Autodesk Inventor part; units mm, degrees
ref_plane "washer_to_base_XY" through (0, -0.48, 0) normal (0, 1, 0) x (1, 0, 0)
ref_plane "washer_to_base_YZ" through (0, -0.48, 0) normal (1, 0, 0) x (0, 0, -1)
ref_plane "washer_to_base_ZX" through (0, -0.48, 0) normal (0, 0, -1) x (0, 1, 0)
sketch "Sketch_1" plane through (0, 0, 0) normal (1, 0, 0) x (0, 1, 0)
  arc A0 (1.4, 9.75) -> (0, 8.35) centre (1.4, 8.35) ccw
  line L0 (0, 8.35) -> (0, -8.35)
  arc A1 (0, -8.35) -> (1.4, -9.75) centre (1.4, -8.35) ccw
  line L1 (1.4, -9.75) -> (16.2, -9.75)
  line L2 (16.2, -9.75) -> (16.2, -8.97)
  line L3 (16.2, -8.97) -> (0.7, -8.97)
  line L4 (0.7, -8.97) -> (0.7, 8.97)
  line L5 (0.7, 8.97) -> (16.2, 8.97)
  line L6 (16.2, 8.97) -> (16.2, 9.75)
  line L7 (16.2, 9.75) -> (1.4, 9.75)
extrude "Extrusion1" add sketch "Sketch_1" along normal mid plane 29.8667
sketch "Sketch_3" plane through (0, 0, 9.75) normal (0, 0, 1) x (1, 0, 0)
  line L0 (-22, 25) -> (-22, 0)
  line L1 (-22, 0) -> (-10.85, 0)
  line L2 (-10.85, 0) -> (-10.85, 0.7)
  line L3 (-10.85, 0.7) -> (-12.7818, 13.6261)
  arc A0 (-12.7301, 13.9322) -> (-12.7818, 13.6261) centre (-12.2873, 13.7) ccw
  line L4 (-12.7301, 13.9322) -> (-8.2588, 12.7341)
  arc A1 (-8.2588, 12.7341) -> (-7, 13.7) centre (-8, 13.7) ccw
  line L5 (-7, 13.7) -> (-7, 15.2)
  arc A2 (-5, 15.2) -> (-7, 15.2) centre (-6, 15.2) ccw
  line L6 (-5, 15.2) -> (-5, 0)
  line L7 (-5, 0) -> (5, 0)
  line L8 (5, 0) -> (5, 14.7)
  arc A3 (8, 14.7) -> (5, 14.7) centre (6.5, 14.7) ccw
  line L9 (8, 14.7) -> (8, 13.7)
  arc A4 (8, 13.7) -> (9.3545, 12.765) centre (9, 13.7) ccw
  line L10 (9.3545, 12.765) -> (13.1394, 14.2)
  arc A5 (13.6339, 13.6264) -> (13.1394, 14.2) centre (13.1394, 13.7) ccw
  line L11 (13.6339, 13.6264) -> (11.6047, 0)
  line L12 (11.6047, 0) -> (22, 0)
  line L13 (22, 0) -> (22, 25)
  line L14 (22, 25) -> (-22, 25)
extrude "Extrusion2" cut sketch "Sketch_3" against normal blind 1.4
sketch "Sketch_2" plane through (0, 0, -9.75) normal (0, 0, 1) x (1, 0, 0)
  line L0 (-22, 25) -> (-22, 0)
  line L1 (-22, 0) -> (-10.85, 0)
  line L2 (-10.85, 0) -> (-10.85, 0.7)
  line L3 (-10.85, 0.7) -> (-12.7818, 13.6261)
  arc A0 (-12.7301, 13.9322) -> (-12.7818, 13.6261) centre (-12.2873, 13.7) ccw
  line L4 (-12.7301, 13.9322) -> (-8.2588, 12.7341)
  arc A1 (-8.2588, 12.7341) -> (-7, 13.7) centre (-8, 13.7) ccw
  line L5 (-7, 13.7) -> (-7, 15.2)
  arc A2 (-5, 15.2) -> (-7, 15.2) centre (-6, 15.2) ccw
  line L6 (-5, 15.2) -> (-5, 0)
  line L7 (-5, 0) -> (5, 0)
  line L8 (5, 0) -> (5, 14.7)
  arc A3 (8, 14.7) -> (5, 14.7) centre (6.5, 14.7) ccw
  line L9 (8, 14.7) -> (8, 13.7)
  arc A4 (8, 13.7) -> (9.3545, 12.765) centre (9, 13.7) ccw
  line L10 (9.3545, 12.765) -> (13.1394, 14.2)
  arc A5 (13.6339, 13.6264) -> (13.1394, 14.2) centre (13.1394, 13.7) ccw
  line L11 (13.6339, 13.6264) -> (11.6047, 0)
  line L12 (11.6047, 0) -> (22, 0)
  line L13 (22, 0) -> (22, 25)
  line L14 (22, 25) -> (-22, 25)
extrude "Extrusion3" cut sketch "Sketch_2" along normal blind 1.4
sketch "Sketch4" plane through (-5, 0, 8.35) normal (0, -1, 0) x (1, 0, 0)
  point P0 (5, -8.35)
hole "Hole1" at (0, 0, 0) direction (0, 1, 0) diameter 10.5 depth 1
sketch "Sketch_5" plane through (0, 0, 0) normal (0, 0, 1) x (1, 0, 0)
  line L0 (-15.85, 1) -> (-15.85, -1)
  line L1 (-15.85, -1) -> (15.62, -1)
  line L2 (15.62, -1) -> (15.62, 1)
  line L3 (15.62, 1) -> (12.12, 1)
  line L4 (12.12, 1) -> (12.12, 0)
  line L5 (12.12, 0) -> (-10.85, 0)
  line L6 (-10.85, 0) -> (-10.85, 1)
  line L7 (-10.85, 1) -> (-15.85, 1)
extrude "Extrusion4" cut sketch "Sketch_5" along normal mid plane 16.7
sketch "Sketch_9" plane through (0, 0, 9.75) normal (0, 0, 1) x (1, 0, 0)
  line L0 (11.6047, 0) -> (22, 0)
  line L1 (22, 0) -> (22, 25)
  line L2 (22, 25) -> (15.3276, 25)
  line L3 (15.3276, 25) -> (11.6047, 0)
extrude "Extrusion5" cut sketch "Sketch_9" against normal blind 19.5
sketch "Sketch_6" plane through (-10.85, 0, 0) normal (1, 0, 0) x (0, 0, -1)
  arc A0 (-8.265, -7.8) -> (-6.765, -9.3) centre (-6.765, -7.8) ccw
  line L0 (-6.765, -9.3) -> (6.765, -9.3)
  arc A1 (6.765, -9.3) -> (8.265, -7.8) centre (6.765, -7.8) ccw
  line L1 (8.265, -7.8) -> (8.265, 0.7)
  line L2 (8.265, 0.7) -> (-8.265, 0.7)
  line L3 (-8.265, 0.7) -> (-8.265, -7.8)
extrude "Extrusion6" add sketch "Sketch_6" along normal blind 0.7
sketch "Sketch_7" plane through (0, 0, 0) normal (0, 0, 1) x (1, 0, 0)
  line L0 (10.8547, -3.3) -> (11.5547, -3.3)
  line L1 (11.5547, -3.3) -> (11.5547, -0.3252)
  line L2 (11.5547, -0.3252) -> (11.6047, 0)
  line L3 (11.6047, 0) -> (11.6047, 0.7)
  line L4 (11.6047, 0.7) -> (10.8547, 0.7)
  line L5 (10.8547, 0.7) -> (10.8547, -3.3)
extrude "Extrusion7" add sketch "Sketch_7" along normal mid plane 2.5
sketch "Sketch_8" plane through (11.555, 0, 0) normal (1, 0, 0) x (0, 0, -1)
  line L0 (-1.5, -0.5) -> (-1.5, -4.5)
  line L1 (-1.5, -4.5) -> (1.5, -4.5)
  line L2 (1.5, -4.5) -> (1.5, -0.5)
  line L3 (1.5, -0.5) -> (1.25, -0.5)
  line L4 (1.25, -0.5) -> (1.25, -2.8)
  arc A0 (0.75, -3.3) -> (1.25, -2.8) centre (0.75, -2.8) ccw
  line L5 (0.75, -3.3) -> (-0.75, -3.3)
  arc A1 (-1.25, -2.8) -> (-0.75, -3.3) centre (-0.75, -2.8) ccw
  line L6 (-1.25, -2.8) -> (-1.25, -0.5)
  line L7 (-1.25, -0.5) -> (-1.5, -0.5)
extrude "Extrusion8" cut sketch "Sketch_8" against normal blind 0.78
ref_plane "washer_to_base_XY" through (0, -0.48, 0) normal (0, 1, 0) x (1, 0, 0)
ref_plane "washer_to_base_YZ" through (0, -0.48, 0) normal (1, 0, 0) x (0, 0, -1)
ref_plane "washer_to_base_ZX" through (0, -0.48, 0) normal (0, 0, -1) x (0, 1, 0)
ref_plane "washer_to_insert_XY" through (0, 0.7, 0) normal (0, 1, 0) x (1, 0, 0)
ref_plane "washer_to_insert_YZ" through (0, 0.7, 0) normal (1, 0, 0) x (0, 0, -1)
ref_plane "washer_to_insert_ZX" through (0, 0.7, 0) normal (0, 0, -1) x (0, 1, 0)
properties part number "lock_washer_na"
Build history of the part. All positions in model axes, mm. A direction names the side the tool comes from. Round coordinates to 2 decimals unless told otherwise and drop trailing zeros. Order: outer loops, then holes, each group sorted by start corner. A loop starts at its lowest first (then second) coordinate and runs counter-clockwise, first axis right, second up. Notation, with made-up numbers: (-6.5, 11.25) - (41.5, 11.25) arc R14 ccw to (41.5, 30.25) - close; hole circle Ø2 at (52, 25). An arc over 180 degrees is marked (long way). Use a Markdown table: item, result.
1) Saw through at C-C on y = 5. Write the cut outline in (x, z).
Recorded:
| item | result |
|---|---|
| outline | (-11.49, -9.75) - (-5, -9.75) - (-5, -8.97) - (-11.49, -8.97) - close; (-11.49, 8.97) - (-5, 8.97) - (-5, 9.75) - (-11.49, 9.75) - close; (5, -9.75) - (12.35, -9.75) - (12.35, -8.97) - (5, -8.97) - close; (5, 8.97) - (12.35, 8.97) - (12.35, 9.75) - (5, 9.75) - close |
2) Pull direction X, two halves, no side cores. Call faces 1 (the face through (-8, 7, 9.75)), 2 (the face through (11.555, -2, 0)), 3 (the face through (5, 7.2, -9.4)), 4 (the face through (8.4, 12.9, -9.4)): pulls with the +X half, pulls with the -X half, needs draft (parallel to the pull), parting line crosses it, or undercut.
Recorded:
| item | result |
|---|---|
| face 1 | needs draft |
| face 2 | pulls with the +X half |
| face 3 | undercut |
| face 4 | undercut |
3) Saw through at B-B on x = 0. Write the cut outline in (y, z), and give its area (3 significant figures).
Recorded:
| item | result |
|---|---|
| outline | (0, -8.35) - (0.7, -8.35) - (0.7, -5.25) - (0, -5.25) - close; (0, 5.25) - (0.7, 5.25) - (0.7, 8.35) - (0, 8.35) - close |
| area | 4.34 mm² |
4) Tool access for faces 5 (the face through (-8, 8, 8.97)), 6 (the face through (10.855, -2, 0)), 7 (the face through (11.22, 13.472, 9.365)), 8 (the face through (8, 9, 9.75)): list every direction of +Z, -Z, +X, -X, +Y, -Y with a clear straight run to the whole face (end or side of a thin tool).
Recorded:
| item | result |
|---|---|
| face 5 | +X, -X, +Y |
| face 6 | +Z, -Z, -Y |
| face 7 | +Z, -Z, +Y |
| face 8 | +Z, +X, -X, +Y, -Y |
5) Flat gauge pins, fed straight in: pin 1 Ø1.5 at (y, z) = (-5, 0.5) entering from -X; pin 2 Ø0.9 at (y, z) = (14.5, 9.5) entering from +X; pin 3 Ø0.8 at (x, y) = (-10.5, -3) entering from -Z (3 decimals). Where does each tip first touch, or does it go through?
Recorded:
| item | result |
|---|---|
| pin 1 | stops at x = -10.85 |
| pin 2 | stops at x = 13.5 |
| pin 3 | stops at z = -8.265 |
6) Wall check: L1, parallel to Z at x = 0, y = 0.4; L2, parallel to Z at x = -7.5, y = 11.75; L3, parallel to Y at x = 11, z = 0.75. Give the ranges that are in metal, low to high.
Recorded:
| item | result |
|---|---|
| L1 | z = -8.35 to -5.25, 5.25 to 8.35 |
| L2 | z = -9.75 to -8.97, 8.97 to 9.75 |
| L3 | y = -3.3 to 0.7 |
7) Saw through at A-A on z = 0. Write the cut outline in (x, y).
Recorded:
| item | result |
|---|---|
| outline | (-10.85, -9.3) - (-10.15, -9.3) - (-10.15, 0) - (-5.25, 0) - (-5.25, 0.7) - (-10.85, 0.7) - close; (5.25, 0) - (10.85, 0) - (10.85, -3.3) - (11.55, -3.3) - (11.55, -0.33) - (11.6, 0) - (11.71, 0.7) - (5.25, 0.7) - close |
8) Saw through at D-D on y = 13.25. Give the number of separate pieces and of enclosed holes in the cut face, and give its area (3 significant figures).
Recorded:
| item | result |
|---|---|
| separate pieces | 8 |
| enclosed holes | 0 |
| area | 16.7 mm² |
